Read the model definition and answer for the solid it produces. Units are mm, in the model's axes. Face numbers are marked on the shaded views. A direction names the side the tool comes from. Round coordinates to 2 decimals unless told otherwise and drop trailing zeros. Order: outer loops, then holes, each group sorted by start corner. A loop starts at its lowest first (then second) coordinate and runs counter-clockwise, first axis right, second up. Notation, with made-up numbers: (53.25, 62) -> (76.25, 62) arc R23 ccw to (76.25, 101) -> close; hole circle Ø4 at (24, -18.5). An arc over 180 degrees is marked (long way). One line per item, written item: value. Start each with the question number.
1. Section D-D (x = -27) is taken. Give the vertices of the cut face in (y, z).
2. For the marked faces 4 and 5, determine the directions among +Z, -Z, +X, -X, +Y, -Y from which every point of the face is accessible in a straight line to the end or side of a thin tool.
3. Consider line 1 (Z direction, x = 3, y = 17.5); line 2 (Z direction, x = -7, y = 15.5); line 3 (Y direction, x = 4, z = -28.5). Determine where each line is inside the solid, lowest interval first.
4. Flat-ended cylindrical pins translate along their axes: pin 1 Ø4 at (x, y) = (-35.5, 21.5) entering from -Z; pin 2 Ø1.4 at (x, y) = (-65.5, 21.5) entering from +Z; pin 3 Ø10 at (x, y) = (-53, 18.5) entering from +Z; pin 4 Ø14 at (x, y) = (-3.5, 22) entering from +Z (3 decimals). Find the tip coordinate at first contact, or state that the pin passes through.
5. The mould has two halves that part along Z. Classify the marked faces 1, 2 and 3: released by +Z, released by -Z, zero draft, split by the parting line, or undercut.
6. Section A-A (y = 16.25) is taken. Give the vertices of the cut face in (x, z) (3 decimals), then the cut area to 3 significant figures.
7. Section B-B (x = 0) is taken. Give the vertices of the cut face in (y, z) (3 decimals).
8. Section C-C (z = -8) is taken. Give the vertices of the cut face in (x, y), then the cut area to 3 significant figures.
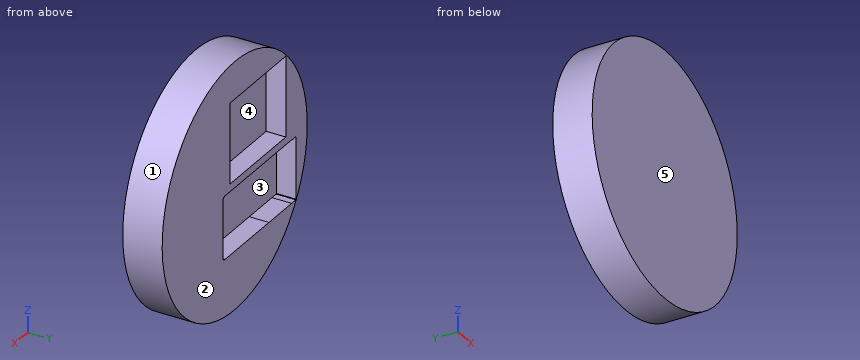
from build123d import *

# Parameters (mm, degrees)
SKETCH1_R           = 79.375
BOSS_EXTRUDE1_DEPTH = 25.4
CUT_EXTRUDE1_DEPTH  = 12.7


with BuildPart() as part:
    # Sketch1 → Boss-Extrude1 (new body)
    with BuildSketch(Plane(origin=(0, 0, 0), x_dir=(1, 0, 0), z_dir=(0, 1, 0))):
        with Locations(Location((0, 0, 0), (0, 0, 270))):
            Circle(SKETCH1_R)
    extrude(amount=BOSS_EXTRUDE1_DEPTH)

    # Sketch2 → Cut-Extrude1 (cut)
    with BuildSketch(Plane(origin=(0, 25.4, 0), x_dir=(1, 0, 0), z_dir=(0, 1, 0))):
        Polygon((4.96096917, -3.583661606), (4.96096917, -7.48907527), (4.96096917, -8.37807527), (4.96096917, -50.554447942), (4.96096917, -51.443447942), (4.96096917, -55.348861606), (-55.99903083, -55.348861606), (-55.99903083, -51.443447942), (-55.99903083, -50.554447942), (-55.99903083, -8.37807527), (-55.99903083, -7.48907527), (-55.99903083, -3.583661606), align=None)
        with BuildLine():
            Line((13.069814764, 39.393138394), (13.069814764, 3.833138394))
            ThreePointArc((13.069814764, 3.833138394), (12.325865988, 2.03708717), (10.529814764, 1.293138394))
            Line((10.529814764, 1.293138394), (-37.221874349, 1.293138394))
            Line((-37.221874349, 1.293138394), (-37.475874266, 1.293138394))
            Line((-37.475874266, 1.293138394), (-62.366588392, 1.293138394))
            Line((-62.366588392, 1.293138394), (-62.426979393, 1.547138394))
            Line((-62.426979393, 1.547138394), (-67.193874266, 1.547138394))
            Line((-67.193874266, 1.547138394), (-67.193874266, 16.202925843))
            Line((-67.193874266, 16.202925843), (-67.193874266, 27.023351013))
            Line((-67.193874266, 27.023351013), (-67.193874266, 41.679138428))
            Line((-67.193874266, 41.679138428), (-66.939875034, 41.933134494))
            Line((-66.939875034, 41.933134494), (-62.366588392, 41.9331351))
            Line((-62.366588392, 41.9331351), (-37.475874266, 41.933138394))
            Line((-37.475874266, 41.933138394), (-37.221874349, 41.933138394))
            Line((-37.221874349, 41.933138394), (10.529814764, 41.933138394))
            ThreePointArc((10.529814764, 41.933138394), (12.325865988, 41.189189618), (13.069814764, 39.393138394))
        make_face()
    extrude(amount=-CUT_EXTRUDE1_DEPTH, mode=Mode.SUBTRACT)


solid = part.part
Answer:
1. outline: (0, -74.64) -> (25.4, -74.64) -> (25.4, -41.93) -> (12.7, -41.93) -> (12.7, -1.29) -> (25.4, -1.29) -> (25.4, 3.58) -> (12.7, 3.58) -> (12.7, 55.35) -> (25.4, 55.35) -> (25.4, 74.64) -> (0, 74.64) -> close
2. face 4: +Y
2. face 5: +Z, -Z, +X, -X, -Y
3. line 1: -79.32 to -41.93, -1.29 to 3.58, 55.35 to 79.32
3. line 2: -79.07 to -41.93, -1.29 to 3.58, 55.35 to 79.07
3. line 3: 0 to 12.7
4. pin 1: z = -71.96
4. pin 2: z = 45.84
4. pin 3: z = 63.22
4. pin 4: z = 79.375
5. face 1: split by the parting line
5. face 2: zero draft
5. face 3: undercut
6. outline: circle Ø158.75 at (0, 0); hole (-67.194, -41.679) -> (-66.94, -41.933) -> (-37.476, -41.933) -> (10.53, -41.933) arc R2.54 ccw to (13.07, -39.393) -> (13.07, -3.833) arc R2.54 ccw to (10.53, -1.293) -> (-62.367, -1.293) -> (-62.427, -1.547) -> (-67.194, -1.547) -> close; hole (-55.999, 3.584) -> (4.961, 3.584) -> (4.961, 55.349) -> (-55.999, 55.349) -> close
6. area: 13,400 mm^2
7. outline: (0, -79.375) -> (25.4, -79.375) -> (25.4, -41.933) -> (12.7, -41.933) -> (12.7, -1.293) -> (25.4, -1.293) -> (25.4, 3.584) -> (12.7, 3.584) -> (12.7, 55.349) -> (25.4, 55.349) -> (25.4, 79.375) -> (0, 79.375) -> close
8. outline: (-78.97, 0) -> (78.97, 0) -> (78.97, 25.4) -> (13.07, 25.4) -> (13.07, 12.7) -> (-67.19, 12.7) -> (-67.19, 25.4) -> (-78.97, 25.4) -> close
8. area: 2,990 mm^2
